from build123d import *

# Parameters (mm, degrees)
BOSS_EXTRUDE1_DEPTH = 80
SKETCH3_R           = 3
CUT_EXTRUDE1_DEPTH  = 26


with BuildPart() as part:
    # Sketch1 → Boss-Extrude1 (new body)
    with BuildSketch(Plane(origin=(0, 0, 0), x_dir=(1, 0, 0), z_dir=(0, 1, 0))):
        with BuildLine():
            Line((11.25, 13.25), (-11.25, 13.25))
            ThreePointArc((-11.25, 13.25), (-12.664213562, 12.664213562), (-13.25, 11.25))
            Line((-13.25, 11.25), (-13.25, -8.25))
            ThreePointArc((-13.25, -8.25), (-12.664213562, -9.664213562), (-11.25, -10.25))
            Line((-11.25, -10.25), (-10.25, -10.25))
            Line((-10.25, -10.25), (-10.25, 10.25))
            Line((-10.25, 10.25), (10.25, 10.25))
            Line((10.25, 10.25), (10.25, -10.25))
            Line((10.25, -10.25), (11.25, -10.25))
            ThreePointArc((11.25, -10.25), (12.664213562, -9.664213562), (13.25, -8.25))
            Line((13.25, -8.25), (13.25, 11.25))
            ThreePointArc((13.25, 11.25), (12.664213562, 12.664213562), (11.25, 13.25))
        make_face()
    extrude(amount=BOSS_EXTRUDE1_DEPTH)

    # Sketch3 → Cut-Extrude1 (cut)
    with BuildSketch(Plane(origin=(0, 0, -13.25), x_dir=(-1, 0, 0), z_dir=(0, 0, -1))):
        with Locations((0, 70)):
            Circle(SKETCH3_R)
        with Locations((0, 10)):
            Circle(SKETCH3_R)
    extrude(amount=-CUT_EXTRUDE1_DEPTH, mode=Mode.SUBTRACT)


solid = part.part
For this review, take the finished solid that the model builds, in its own axes (mm). A direction names the side the tool comes from. Give positions to 0.01 mm unless a question says otherwise; leave off trailing zeros. Loops run counter-clockwise (first coordinate to the right, second up) from the corner with the lowest first, then second, coordinate; pieces in that order, holes last.
Item 1: Take a section at B-B, the plane x = 0. State the section outline as (y, z) points.
Item 2: Take a section at C-C, the plane z = -5.75. State the section outline as (x, y) points, and give its area (3 significant figures).
Item 3: Take a section at A-A, the plane y = 70. State the section outline as (x, z) points.
Item 4: For line 1 along Y through (x, z) = (0, -11.05); line 2 along X through (y, z) = (10.5, -8); line 3 along Z through (x, y) = (-0.75, 73), list the stretches that pass through material, from the lowest coordinate up.
Item 5: Draft analysis for pull direction Y (two halves, no side actions). For faces 3 (the cylindrical face through (-12.68, 39.44, 9.65)), 4 (the cylindrical face through (3, 10, -12)), 5 (the flat face through (-1, 80, -11)), state which applies: +Y half, -Y half, draft (parallel to the pull), parting line (faces both ways), or undercut.
Item 6: Take a section at D-D, the plane y = 60.5. State the section outline as (x, z) points, and give its area (3 significant figures).
Item 7: Tool access review of faces 1 (the flat face through (-10.25, 39, 0)), 2 (the flat face through (-1, 0, -11)): name each direction out of +Z, -Z, +X, -X, +Y, -Y from which nothing blocks a thin tool from reaching the whole face with its end or side.
Item 8: Insertion check: pin 1 (5 mm diameter, centred on x = 0, y = 70, fed in from +Z). The pin has a flat end and moves straight along its axis. Give the tip position at first contact, or say it passes through.
Calculated:
1. outline: (0, -13.25) - (7, -13.25) - (7, -10.25) - (0, -10.25) - close; (13, -13.25) - (67, -13.25) - (67, -10.25) - (13, -10.25) - close; (73, -13.25) - (80, -13.25) - (80, -10.25) - (73, -10.25) - close
2. outline: (-13.25, 0) - (-10.25, 0) - (-10.25, 80) - (-13.25, 80) - close; (10.25, 0) - (13.25, 0) - (13.25, 80) - (10.25, 80) - close
2. area: 480 mm2
3. outline: (-13.25, -11.25) arc R2 ccw to (-11.25, -13.25) - (-3, -13.25) - (-3, -10.25) - (-10.25, -10.25) - (-10.25, 10.25) - (-11.25, 10.25) arc R2 ccw to (-13.25, 8.25) - close; (3, -13.25) - (11.25, -13.25) arc R2 ccw to (13.25, -11.25) - (13.25, 8.25) arc R2 ccw to (11.25, 10.25) - (10.25, 10.25) - (10.25, -10.25) - (3, -10.25) - close
4. line 1: y = 0 to 7, 13 to 67, 73 to 80
4. line 2: x = -13.25 to -10.25, 10.25 to 13.25
4. line 3: z = -13.25 to -10.25
5. face 3: draft
5. face 4: undercut
5. face 5: +Y half
6. outline: (-13.25, -11.25) arc R2 ccw to (-11.25, -13.25) - (11.25, -13.25) arc R2 ccw to (13.25, -11.25) - (13.25, 8.25) arc R2 ccw to (11.25, 10.25) - (10.25, 10.25) - (10.25, -10.25) - (-10.25, -10.25) - (-10.25, 10.25) - (-11.25, 10.25) arc R2 ccw to (-13.25, 8.25) - close
6. area: 199 mm2
7. face 1: +Z, +Y, -Y
7. face 2: +Z, -Z, +X, -X, -Y
8. pin 1: passes through
